Model file for the job. Use its own axes, mm. Round coordinates to 2 decimals unless told otherwise and drop trailing zeros. Order: outer loops, then holes, each group sorted by start corner. A loop starts at its lowest first (then second) coordinate and runs counter-clockwise, first axis right, second up. Notation, with made-up numbers: (85.5, 28) -> (117.5, 28) arc R25 ccw to (117.5, 58) -> close; hole circle Ø6 at (-18, -35.5). An arc over 180 degrees is marked (long way). Use CSV: the item, a comma, the result in double quotes.
```python
from build123d import *

# Parameters (mm, degrees)
SKETCH1_W                      = 69.85
SKETCH1_H                      = 19.05
BOSS_EXTRUDE1_DEPTH            = 19.05
F_3_8_CLEARANCE_HOLE1_D        = 9.8044
F_5_16_0_3125_DIAMETER_HOLE1_D = 7.9375


with BuildPart() as part:
    # Sketch1 → Boss-Extrude1 (new body)
    with BuildSketch(Plane.XY):
        Rectangle(SKETCH1_W, SKETCH1_H)
    extrude(amount=BOSS_EXTRUDE1_DEPTH)

    # 3/8 Clearance Hole1 (through all)
    with Locations(Plane.XY.offset(19.05)):
        with Locations((0, 0)):
            Hole(F_3_8_CLEARANCE_HOLE1_D / 2)

    # 5/16 (0.3125) Diameter Hole1 (through all)
    with Locations(Plane(origin=(0, 9.525, 0), x_dir=(1, 0, 0), z_dir=(0, 1, 0))):
        with Locations((-25.4, -9.525), (25.4, -9.525)):
            Hole(F_5_16_0_3125_DIAMETER_HOLE1_D / 2)


solid = part.part
```
Q1. Cut at B-B (x = 0). Give the cut face in (y, z) (3 decimals).
From the geometry:
outline,"(-9.525, 0) -> (-4.902, 0) -> (-4.902, 19.05) -> (-9.525, 19.05) -> close; (4.902, 0) -> (9.525, 0) -> (9.525, 19.05) -> (4.902, 19.05) -> close"
Q2. Mould opens along X. For faces 1 (the cylindrical face through (-21.435, -0.133, 9.351)), 2 (the flat face through (0, 6, 0)), 3 (the flat face through (34.925, 0, 9)) say: +X half, -X half, draft (parallel to the pull), parting line (faces both ways), or undercut.
From the geometry:
face 1,"undercut"
face 2,"draft"
face 3,"+X half"
Q3. Probe line 1 along X through (y, z) = (0.25, 4.25) (3 decimals); line 2 along X through (y, z) = (-5.25, 13) (3 decimals); line 3 along X through (y, z) = (-6.25, 6) (3 decimals). List the from-to ranges inside material, lowest first.
From the geometry:
line 1,"x = -34.925 to -4.896, 4.896 to 34.925"
line 2,"x = -34.925 to -27.317, -23.483 to 23.483, 27.317 to 34.925"
line 3,"x = -34.925 to -27.224, -23.576 to 23.576, 27.224 to 34.925"
Q4. Cut at A-A (y = 0). State how many separate pieces and enclosed holes the cut face has, plus the area to 3 significant figures.
From the geometry:
separate pieces,"2"
enclosed holes,"2"
area,"1,040 mm²"
Q5. Pin check, flat tip, straight feed: pin 1 (7 mm diameter, centred on x = 25.4, z = 9.525, fed in from +Y). Stop position of the tip, or through.
From the geometry:
pin 1,"passes through"
Q6. Cut at C-C (z = 11.5). Give the cut face in (x, y) (3 decimals).
From the geometry:
outline,"(-34.925, -9.525) -> (-28.842, -9.525) -> (-28.842, 9.525) -> (-34.925, 9.525) -> close; (-21.958, -9.525) -> (21.958, -9.525) -> (21.958, 9.525) -> (-21.958, 9.525) -> close; (28.842, -9.525) -> (34.925, -9.525) -> (34.925, 9.525) -> (28.842, 9.525) -> close; hole circle Ø9.804 at (0, 0)"
